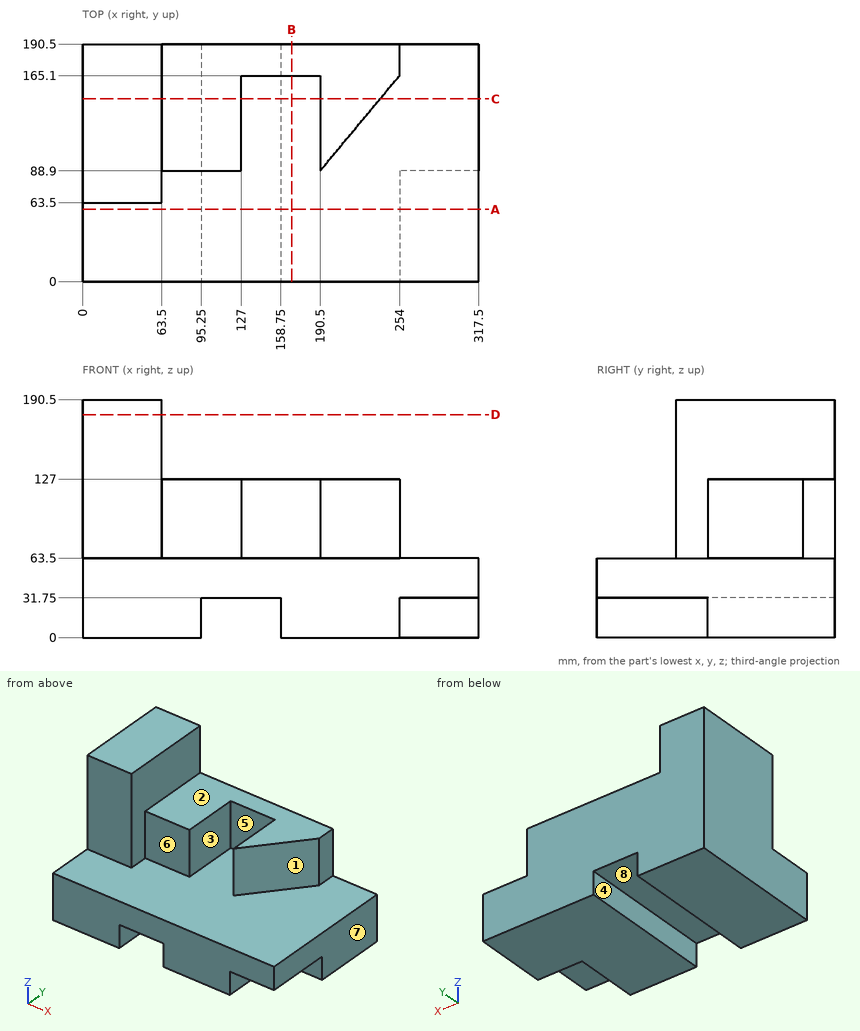
Verification items for this drawing (mm, ordinates from the low corner). A direction names the side the tool comes from. Coordinates: 2 decimals unless noted, no trailing zeros. Write each loop counter-clockwise with the first axis right and the second up, starting at its lowest first coordinate (ties: lowest second). Pieces come first, ordered by that corner, then holes. Notation, with made-up numbers: (-10, -13.75) -> (11, -13.75) arc R26 cw to (11, 12.25) -> close; hole circle Ø3 at (85.25, 81.25). An arc over 180 degrees is marked (long way). Use CSV: the item, a comma, the result in double quotes. Start each with the question number.
Item 1: Mould release check, pull along X, two halves, no side actions. Record for the marked faces 5, 6, 7 and 8: released by +X, released by -X, zero draft, split by the parting line, or undercut.
Item 2: Cross-section at B-B, the plane x = 167.5. Record the cut outline in (y, z), plus the area to 3 significant figures.
Item 3: Depth check by flat-ended pin: pin 1 Ø6 at (x, y) = (65, 48.5) entering from +Z; pin 2 Ø19 at (x, z) = (158.5, 79.5) entering from -Y; pin 3 Ø8 at (y, z) = (89.5, 152.5) entering from +X. Enter the tip coordinate at first touch or a pass-through.
Item 4: Thickness scan on line 1 (X direction, y = 175.5, z = 19); line 2 (X direction, y = 111.5, z = 75.5); line 3 (Y direction, x = 89.5, z = 75). Record the ranges inside material, lowest first.
Item 5: Cross-section at A-A, the plane y = 58. Record the cut outline in (x, z).
Item 6: Cross-section at D-D, the plane z = 178.5. Record the cut outline in (x, y).
Item 7: Set-up check for the marked faces 1, 2, 3 and 4: record each of +Z, -Z, +X, -X, +Y, -Y from which the full face is reachable in a straight line by a thin tool's end or side.
Item 8: Cross-section at C-C, the plane y = 146.5. Record the cut outline in (x, z), plus the area to 3 significant figures.
Answers:
1,face 5,"undercut"
1,face 6,"zero draft"
1,face 7,"released by +X"
1,face 8,"undercut"
2,outline,"(0, 0) -> (190.5, 0) -> (190.5, 127) -> (165.1, 127) -> (165.1, 63.5) -> (0, 63.5) -> close"
2,area,"13,700 mm^2"
3,pin 1,"z = 63.5"
3,pin 2,"y = 165.1"
3,pin 3,"x = 63.5"
4,line 1,"0 to 95.25, 158.75 to 317.5"
4,line 2,"0 to 127, 190.5 to 209.33"
4,line 3,"88.9 to 190.5"
5,outline,"(0, 0) -> (95.25, 0) -> (95.25, 31.75) -> (158.75, 31.75) -> (158.75, 0) -> (254, 0) -> (254, 31.75) -> (317.5, 31.75) -> (317.5, 63.5) -> (0, 63.5) -> close"
6,outline,"(0, 63.5) -> (63.5, 63.5) -> (63.5, 190.5) -> (0, 190.5) -> close"
7,face 1,"+Z, +X, -Y"
7,face 2,"+Z, +X, +Y, -Y"
7,face 3,"+Z, -Y"
7,face 4,"-Z, +Y, -Y"
8,outline,"(0, 0) -> (95.25, 0) -> (95.25, 31.75) -> (158.75, 31.75) -> (158.75, 0) -> (317.5, 0) -> (317.5, 63.5) -> (238.5, 63.5) -> (238.5, 127) -> (190.5, 127) -> (190.5, 63.5) -> (127, 63.5) -> (127, 127) -> (63.5, 127) -> (63.5, 190.5) -> (0, 190.5) -> close"
8,area,"33,300 mm^2"
